For this review, take the finished solid that the model builds, in its own axes (mm). A direction names the side the tool comes from. Round coordinates to 2 decimals unless told otherwise and drop trailing zeros. Write each loop counter-clockwise with the first axis right and the second up, starting at its lowest first coordinate (ties: lowest second). Pieces come first, ordered by that corner, then holes. Notation, with made-up numbers: M 65,-19.75 L 101,-19.75 A17 cw 101,-9.75 Z; hole C 39.25,6.25 d1. An arc over 180 degrees is marked long. Answer in a Markdown table with one row per item.
```python
from build123d import *

# Parameters (mm, degrees)
F0_R     = 14.3848333842
F1_DEPTH = 17.3482
F4_R     = 2.159
F5_DEPTH = 1.016
F6_D     = 2.7051
F6_DEPTH = 5.87375
F6_TIP   = 0.8126940303
F8_D     = 2.5


# Not quite as in the source:
# - a feature names something its author has since deleted; it is built from what else it names


with BuildPart() as f1:
    # F0 (on Top) → F1 (new body)
    with BuildSketch(Plane.XY):
        Circle(F0_R)
    extrude(amount=F1_DEPTH)

    # F4 (on face) → F5 (join)
    with BuildSketch(Plane.XY.offset(17.3482)):
        Circle(F4_R)
    extrude(amount=F5_DEPTH)

    # F6
    with Locations(Plane.XY.offset(17.3482)):
        with Locations((0, 9.0678), (0, -9.0678)):
            Hole(F6_D / 2, depth=F6_DEPTH)
            with Locations((0, 0, -(F6_DEPTH + F6_TIP / 2))):  # 118° drill point
                Cone(0, F6_D / 2, F6_TIP, mode=Mode.SUBTRACT)

    # F8 (through all)
    with Locations(Plane.XY.offset(18.3642)):
        with Locations((0, 0)):
            Hole(F8_D / 2)


solid = f1.part
```
Q1. Mouldability with a two-part tool opening along X and no side actions: class faces 1 (the face through (-0.28, 2.14, 17.85)), 2 (the face through (0.29, -10.39, 14.37)), 3 (the face through (0, -3, 17.348)) as +X half, -X half, draft (parallel to the pull), parting line (faces both ways), or undercut.
Found:
| item | result |
|---|---|
| face 1 | parting line |
| face 2 | undercut |
| face 3 | draft |
Q2. Take a section at D-D (x = -5). State the section outline as (y, z) points, then the cut area to 3 significant figures.
Found:
| item | result |
|---|---|
| outline | M -13.49,0 L 13.49,0 L 13.49,17.35 L -13.49,17.35 Z |
| area | 468 mm² |
Q3. Take a section at A-A (y = 0). State the section outline as (x, z) points.
Found:
| item | result |
|---|---|
| outline | M -14.38,0 L -1.25,0 L -1.25,18.36 L -2.16,18.36 L -2.16,17.35 L -14.38,17.35 Z; M 1.25,0 L 14.38,0 L 14.38,17.35 L 2.16,17.35 L 2.16,18.36 L 1.25,18.36 Z |
Q4. For probe 1 along Y at (x, z) = (0, 13.85); probe 2 along Y at (x, z) = (0, 9); probe 3 along Z at (x, y) = (1, 6.25), list the stretches that pass through material, from the lowest coordinate up.
Found:
| item | result |
|---|---|
| probe 1 | -14.38 to -10.42, -7.72 to -1.25, 1.25 to 7.72, 10.42 to 14.38 |
| probe 2 | -14.38 to -1.25, 1.25 to 14.38 |
| probe 3 | 0 to 17.35 |
Q5. Machinability: for faces 4 (the face through (-3.118, -14.043, 8.553)), 5 (the face through (0.293, 7.747, 14.37)), which of the approach directions +Z, -Z, +X, -X, +Y, -Y give a long, thin tool a straight path to every point of the face, cutting with its end or side? Answer none if there is none.
Found:
| item | result |
|---|---|
| face 4 | +Z, -Z |
| face 5 | +Z |
Q6. Insertion check: P1, Ø6, axis at x = -0.5, y = 10, coming from the +Z side; P2, Ø1, axis at x = -7.5, z = 12, coming from the -Y side; P3, Ø2, axis at x = 0, y = -9.07, coming from the +Z side. Each pin has a flat end and moves straight along its axis. Give the tip position at first contact, or say it passes through.
Found:
| item | result |
|---|---|
| P1 | z = 17.35 |
| P2 | y = -12.57 |
| P3 | z = 11.26 |
Q7. Take a section at B-B (z = 8.25). State the section outline as (x, y) points, then the cut area to 3 significant figures.
Found:
| item | result |
|---|---|
| outline | C 0,0 d28.77; hole C 0,0 d2.5 |
| area | 645 mm² |
Q8. Take a section at C-C (z = 13.75). State the section outline as (x, y) points, then the cut area to 3 significant figures.
Found:
| item | result |
|---|---|
| outline | C 0,0 d28.77; hole C 0,-9.07 d2.71; hole C 0,9.07 d2.71; hole C 0,0 d2.5 |
| area | 634 mm² |
